```python
from build123d import *

# Parameters (mm, degrees)
SKETCH_2_W          = 82
SKETCH_2_H          = 6.001237201
EXTRUDE_1_DEPTH     = 60
SKETCH_3_W          = 82
SKETCH_3_H          = 3.004928021
CUT_EXTRUDE_1_DEPTH = 1.5


with BuildPart() as part:
    # Эскиз1 → Повернуть4 (revolve)
    with BuildSketch(Plane(origin=(0, 0, 0), x_dir=(1, 0, 0), z_dir=(0, 1, 0))):
        Polygon((92.65287472, 0), (92.65287472, 18), (90.65287472, 20), (8.65287472, 20), (7.65287472, 19), (7.65287472, 14.750046626), (8.65287472, 13.750046626), (71.629429714, 13.750046626), (71.629429714, 3.430205497), (76.798526349, 0), align=None)
    revolve(axis=Axis((102.994030824, 0, 0), (-1, 0, 0)))

    # Эскиз2 → Бобышка-Вытянуть1 (add)
    with BuildSketch(Plane(origin=(0, 0, 0), x_dir=(1, 0, 0), z_dir=(0, 1, 0))):
        with Locations((49.65287472, 20.004309421)):
            Rectangle(SKETCH_2_W, SKETCH_2_H)
    extrude(amount=EXTRUDE_1_DEPTH)

    # Эскиз3 → Вырез-Вытянуть1 (cut)
    with BuildSketch(Plane.XZ):
        with Locations((49.65287472, -21.50246401)):
            Rectangle(SKETCH_3_W, SKETCH_3_H)
    extrude(amount=-CUT_EXTRUDE_1_DEPTH, mode=Mode.SUBTRACT)


solid = part.part
```
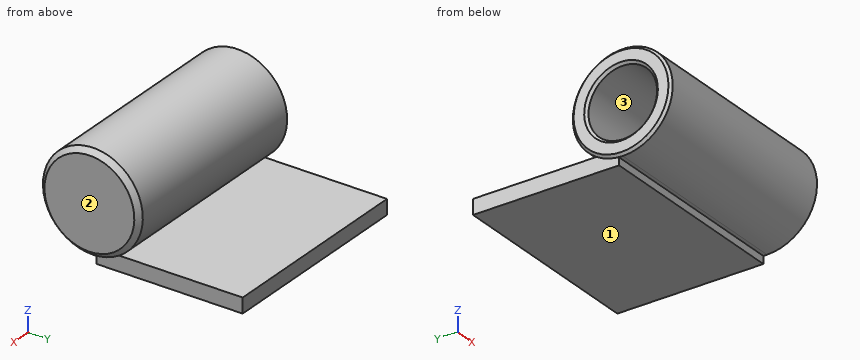
Geometry check sheet. Reference: the model listing, model coordinates, mm. Face numbers are marked on the shaded views. Coordinates: 2 decimals unless noted, no trailing zeros. Write each loop counter-clockwise with the first axis right and the second up, starting at its lowest first coordinate (ties: lowest second). Pieces come first, ordered by that corner, then holes. Notation, with made-up numbers: M 40,58 L 58,58 A19 cw 58,87 Z; hole C -27,88.5 d6. An arc over 180 degrees is marked long. Answer as a JSON object with one key per item and string values.
1. Section check A-A, the plane x = 38. Enter the section's corners in (y, z), plus the area to 3 significant figures.
Answers below:
{"outline": "M 0,-20 L 1.5,-20 L 1.5,-23 L 60,-23 L 60,-17 L 10.53,-17 A20 ccw long Z; hole C 0,0 d27.5", "area": "997 mm²"}
2. Scan lines: L1, parallel to Z at x = 51, y = 0; L2, parallel to Z at x = 42, y = 37. Record each from-to range of solid material in increasing order.
Answers below:
{"L1": "z = -20 to -13.75, 13.75 to 20", "L2": "z = -23 to -17"}
3. Section check B-B, the plane y = 42. Enter the section's corners in (x, z), plus the area to 3 significant figures.
Answers below:
{"outline": "M 8.65,-23 L 90.65,-23 L 90.65,-17 L 8.65,-17 Z", "area": "492 mm²"}
4. Go/stop test with flat-tipped pins: pin 1 Ø1.5 at (x, z) = (62, 1) entering from +Y; pin 2 Ø1.5 at (x, z) = (29.5, -21) entering from -Y; pin 3 Ø10 at (x, z) = (83, -5) entering from -Y; pin 4 Ø0.8 at (x, y) = (57, 1) entering from -Z. Record where each tip stops, or that it passes through.
Answers below:
{"pin 1": "stops at y = 20", "pin 2": "stops at y = 1.5", "pin 3": "stops at y = -20", "pin 4": "stops at z = -20"}
5. Draft check along Z on the marked faces 1, 2 and 3. Enter one of: released by +Z, released by -Z, zero draft, split by the parting line, or undercut.
Answers below:
{"face 1": "released by -Z", "face 2": "zero draft", "face 3": "undercut"}
